Input: part model. Units: mm. Frame: model coordinates. A direction names the side the tool comes from. Coordinates: 2 decimals unless noted, no trailing zeros. Loops run counter-clockwise (first coordinate to the right, second up) from the corner with the lowest first, then second, coordinate; pieces in that order, holes last. Notation, with made-up numbers: (-19.5, 4) -> (31.5, 4) arc R19 ccw to (31.5, 25) -> close; hole circle Ø5 at (21, 89). An arc over 180 degrees is marked (long way). Put each result on its own line as item: value. Start each with the question number.
1) Cut plane C-C (y = 911.25). Return the cut outline in (x, z), plus the area to 3 significant figures.
2) Cut plane B-B (x = 666.5). Return the cut outline in (y, z).
3) Set-up query: faces 1 (the flat face through (673, 913, 1356.675)), 2 (the flat face through (681.91, 916, 1357.56)). Return all of +Z, -Z, +X, -X, +Y, -Y with unobstructed straight access to the full face (end or side cutting, diameter ignored); none if empty.
4) Cut plane D-D (z = 1357.5). Return the cut outline in (x, y), plus the area to 3 significant figures.
5) Pull-direction query (Y, two-part tool) for faces 3 (the flat face through (673, 913, 1336.575)), 4 (the flat face through (676, 905.78, 1347)), 5 (the flat face through (674, 913, 1334.125)), 6 (the flat face through (668, 928.33, 1347)); classes: pulls with the +Y half, pulls with the -Y half, needs draft (parallel to the pull), parting line crosses it, or undercut.
6) Cut plane A-A (z = 1347). Return the cut outline in (x, y).
7) Material intervals for L1, parallel to Y at x = 670.25, z = 1355; L2, parallel to Z at x = 681.5, y = 909.25; L3, parallel to Y at x = 689, z = 1343.25, sorted ascending.
8) Contact query for flat-ended pins moving along their axis: P1, Ø12, axis at y = 919.5, z = 1348.5, coming from the -X side; P2, Ø12, axis at x = 687, z = 1350.5, coming from the +Y side; P3, Ø10, axis at x = 679, z = 1344.5, coming from the +Y side. Output: stop coordinate, or through.
from build123d import *

# Parameters (mm, degrees)
BOSS_EXTRUDE1_START       = 663.104666785
BOSS_EXTRUDE1_OUTLINE_W   = 25
BOSS_EXTRUDE1_OUTLINE_H   = 25
BOSS_EXTRUDE1_OUTLINE_W_2 = 20.1
BOSS_EXTRUDE1_OUTLINE_H_2 = 20.1
BOSS_EXTRUDE1_DEPTH       = 27.857142858
BOSS_EXTRUDE1_START_2     = 1064
BOSS_EXTRUDE1_2_OUTLINE_W = 39
BOSS_EXTRUDE1_2_OUTLINE_H = 25
BOSS_EXTRUDE1_2_DEPTH     = 15.171213372
BOSS_EXTRUDE1_START_3     = 1087.308548084
BOSS_EXTRUDE1_3_OUTLINE_W = 39
BOSS_EXTRUDE1_3_OUTLINE_H = 25
BOSS_EXTRUDE1_3_DEPTH     = 15.691451916
BOSS_EXTRUDE2_DEPTH       = 25
CUT_EXTRUDE2_REACH        = 1648.145
SKETCH7_W                 = 20.1
SKETCH7_H                 = 20.1


with BuildPart() as part:
    # Boss-Extrude1: read off the stored shape, not the designer's step
    # Boss-Extrude1 outline → Boss-Extrude1 (new body)
    with BuildSketch(Plane(origin=(0, 0, 0), x_dir=(0, 0, -1), z_dir=(1, 0, 0)).offset(BOSS_EXTRUDE1_START)):
        with Locations((-1346.624663727, 915.829825752)):
            Rectangle(BOSS_EXTRUDE1_OUTLINE_W, BOSS_EXTRUDE1_OUTLINE_H)
        with Locations((-1346.624663727, 915.829825752)):
            Rectangle(BOSS_EXTRUDE1_OUTLINE_W_2, BOSS_EXTRUDE1_OUTLINE_H_2, mode=Mode.SUBTRACT)
    extrude(amount=BOSS_EXTRUDE1_DEPTH)

    # Boss-Extrude1 2 outline → Boss-Extrude1 2 (cut)
    with BuildSketch(Plane(origin=(0, 0, 0), x_dir=(0.5812381937190959, -0.8137334712067352, 0), z_dir=(0.8137334712067352, 0.5812381937190961, 0)).offset(BOSS_EXTRUDE1_START_2)):
        with Locations((-351.5, -1346.624663727)):
            Rectangle(BOSS_EXTRUDE1_2_OUTLINE_W, BOSS_EXTRUDE1_2_OUTLINE_H)
    extrude(amount=BOSS_EXTRUDE1_2_DEPTH, mode=Mode.SUBTRACT)

    # Boss-Extrude1 3 outline → Boss-Extrude1 3 (cut)
    with BuildSketch(Plane(origin=(0, 0, 0), x_dir=(0.5812381937190959, -0.8137334712067352, 0), z_dir=(0.8137334712067352, 0.5812381937190961, 0)).offset(BOSS_EXTRUDE1_START_3)):
        with Locations((-351.5, -1346.624663727)):
            Rectangle(BOSS_EXTRUDE1_3_OUTLINE_W, BOSS_EXTRUDE1_3_OUTLINE_H)
    extrude(amount=BOSS_EXTRUDE1_3_DEPTH, mode=Mode.SUBTRACT)

    # Sketch5 → Boss-Extrude2 (add)
    with BuildSketch(Plane.XY.offset(1359.124663727)):
        Polygon((663.104666785, 928.329825752), (680.961809643, 903.329825752), (663.104666785, 903.329825752), align=None)
    extrude(amount=-BOSS_EXTRUDE2_DEPTH)

    # Sketch7 → Cut-Extrude2 (cut, up to next)
    with BuildSketch(Plane.ZY.offset(-663.104666785), mode=Mode.PRIVATE) as cut_extrude2_sk1:
        with Locations((1346.624663727, 915.829825752)):
            Rectangle(SKETCH7_W, SKETCH7_H)
    cut_extrude2_tool1 = extrude(cut_extrude2_sk1.sketch, amount=-CUT_EXTRUDE2_REACH, mode=Mode.PRIVATE) & part.part
    add(cut_extrude2_tool1.solids().sort_by_distance((663.104667, 915.829826, 1346.624664))[0], mode=Mode.SUBTRACT)


solid = part.part
Results found:
1. outline: (663.1, 1334.12) -> (685.3, 1334.12) -> (685.3, 1336.57) -> (663.1, 1336.57) -> close; (663.1, 1356.67) -> (685.3, 1356.67) -> (685.3, 1359.12) -> (663.1, 1359.12) -> close
1. area: 109 mm2
2. outline: (903.33, 1334.12) -> (928.33, 1334.12) -> (928.33, 1359.12) -> (903.33, 1359.12) -> close; hole (905.78, 1336.57) -> (925.88, 1336.57) -> (925.88, 1356.67) -> (905.78, 1356.67) -> close
3. face 1: +X, -X
3. face 2: +Z, -Z, +X, +Y
4. outline: (663.1, 903.33) -> (690.96, 903.33) -> (673.1, 928.33) -> (663.1, 928.33) -> close
4. area: 473 mm2
5. face 3: undercut
5. face 4: undercut
5. face 5: needs draft
5. face 6: pulls with the +Y half
6. outline: (663.1, 903.33) -> (690.96, 903.33) -> (689.21, 905.78) -> (663.1, 905.78) -> close; (663.1, 925.88) -> (674.85, 925.88) -> (673.1, 928.33) -> (663.1, 928.33) -> close
7. L1: y = 903.33 to 905.78, 925.88 to 928.33
7. L2: z = 1334.12 to 1336.57, 1356.67 to 1359.12
7. L3: y = 903.33 to 905.78
8. P1: passes through
8. P2: stops at y = 905.78
8. P3: stops at y = 927.08
